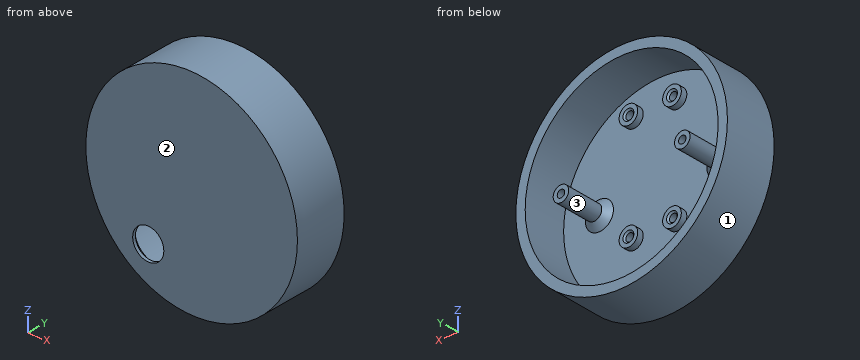
Autodesk Inventor part; units mm, degrees
ref_plane "YZ Plane" through (0, 0, 0) normal (1, 0, 0) x (0, 1, 0)
ref_plane "XZ Plane" through (0, 0, 0) normal (0, 1, 0) x (-1, 0, 0)
ref_plane "XY Plane" through (0, 0, 0) normal (0, 0, 1) x (1, 0, 0)
sketch "Sketch1" plane through (0, 0, 0) normal (0, 1, 0) x (-1, 0, 0)
  circle A0 centre (0, 0) radius 34
  dimension "d0" = 68
extrude "Extrusion1" add sketch "Sketch1" along normal blind 3
sketch "Sketch2" plane through (0, 3, 0) normal (0, 1, 0) x (1, 0, 0)
  circle A0 centre (0, 0) radius 34
  circle A1 centre (0, 0) radius 31
  dimension "d3" = 62
extrude "Extrusion2" add sketch "Sketch2" along normal blind 14
sketch "Sketch3" plane through (0, 3, 0) normal (0, 1, 0) x (1, 0, 0)
  circle A0 centre (0, 0) radius 31
  circle A1 centre (0, 0) radius 19.5
  line L0 (-19.5, 0) -> (19.5, 0)
  circle A2 centre (-19.5, 0) radius 1.2
  circle A3 centre (-19.5, 0) radius 2.5
  circle A4 centre (19.5, 0) radius 1.2
  circle A5 centre (19.5, 0) radius 2.5
  dimension "d6" = 39
  dimension "d7" = 2.4
  dimension "d8" = 5
  dimension "d9" = 2.4
  dimension "d10" = 5
extrude "Extrusion3" add sketch "Sketch3" along normal up to surface (14 mm away) contours A4 L0 A5 A1 | A1 A5 A4 | A1 A5 L0 A4 | A3 L0 A2 A1 | A1 A2 A3 | A1 A2 L0 A3
chamfer "Chamfer1" distance 2 angle 45 2 edges at (-22, 3, 0) (17, 3, 0)
sketch "Sketch4" plane through (0, 3, 0) normal (0, 1, 0) x (1, 0, 0)
  circle A0 centre (-13.9417, 19.5241) radius 5
  dimension "d16" = 10
extrude "Extrusion4" cut sketch "Sketch4" against normal blind 14
chamfer "Chamfer2" distance 2 angle 45 1 edges at (-18.9417, 3, -19.5241)
sketch "Sketch5" plane through (0, 3, 0) normal (0, 1, 0) x (1, 0, 0)
  line L0 (-8.5812, 13.9919) -> (11.4188, 13.9919)
  line L1 (11.4188, 13.9919) -> (11.4188, -26.0081)
  line L2 (11.4188, -26.0081) -> (-8.5812, -26.0081)
  line L3 (-8.5812, -26.0081) -> (-8.5812, 13.9919)
  circle A0 centre (-5.5812, 10.9919) radius 1.25
  circle A1 centre (-5.5812, 10.9919) radius 3
  circle A2 centre (8.4188, 10.9919) radius 1.25
  circle A3 centre (8.4188, 10.9919) radius 3
  circle A4 centre (8.4188, -23.0081) radius 1.25
  circle A5 centre (8.4188, -23.0081) radius 3
  circle A6 centre (-5.5812, -23.0081) radius 1.25
  circle A7 centre (-5.5812, -23.0081) radius 3
  dimension "d22" = 20
  dimension "d23" = 40
  dimension "d24" = 2.5
  dimension "d25" = 6
  dimension "d26" = 2.5
  dimension "d27" = 6
  dimension "d28" = 2.5
  dimension "d29" = 6
  dimension "d30" = 2.5
  dimension "d31" = 6
  dimension "d32" = 3
  dimension "d33" = 3
  dimension "d34" = 3
  dimension "d35" = 3
  dimension "d36" = 3
  dimension "d37" = 3
  dimension "d38" = 3
  dimension "d39" = 3
extrude "Extrusion5" add sketch "Sketch5" along normal blind 2 contours A1 | A3 | A7 | A5
sketch "Sketch6" plane through (-5.5812, 3, -10.9919) normal (0, 1, 0) x (1, 0, 0)
  circle A0 centre (0, 0) radius 1.25
  circle A1 centre (0, 0) radius 1.25
  circle A2 centre (14, 0) radius 1.25
  circle A3 centre (14, -34) radius 1.25
  circle A4 centre (0, -34) radius 1.25
  point P0 (5.5812, -10.9919)
extrude "Extrusion6" cut sketch "Sketch6" against normal blind 2
chamfer "Chamfer3" distance 0.5 angle 45 4 edges at (-6.8312, 5, -10.9919) (7.1688, 5, -10.9919) (-6.8312, 5, 23.0081) (7.1688, 5, 23.0081)
properties part number "obudowa - czujnik dymu"
The model under review builds one solid part; all positions refer to its coordinate system, in mm. Face numbers are marked on the shaded views. Round coordinates to 2 decimals unless told otherwise and drop trailing zeros. Loops run counter-clockwise (first coordinate to the right, second up) from the corner with the lowest first, then second, coordinate; pieces in that order, holes last. Notation, with made-up numbers: (-33.75, 37.25) -> (-16.75, 37.25) arc R10 ccw to (-16.75, 45.25) -> close; hole circle Ø10 at (-12, 89.5). An arc over 180 degrees is marked (long way). Answer as CSV lines item,"result".
1) To check wall thickness, follow line 1 along X through (y, z) = (7.5, 0); line 2 along X through (y, z) = (10, -2); line 3 along Z through (x, y) = (21.5, 16.25). State the ranges of each line that lie inside material, in increasing order. Write a range as from..to.
Geometry results:
line 1,"x = -34..-31, -22..-20.7, -18.3..-17, 17..18.3, 20.7..22, 31..34"
line 2,"x = -33.94..-30.94, -21..-18, 18..21, 30.94..33.94"
line 3,"z = -26.34..-22.33, -1.5..1.5, 22.33..26.34"
2) Add section B-B on z = -5.5. Write out the cut boundary in (x, y), plus the area to 3 significant figures.
Geometry results:
outline,"(-33.55, 0) -> (33.55, 0) -> (33.55, 17) -> (30.51, 17) -> (30.51, 3) -> (-30.51, 3) -> (-30.51, 17) -> (-33.55, 17) -> close"
area,"287 mm²"
3) Add section A-A on y = 6. Write out the cut boundary in (x, z).
Geometry results:
outline,"circle Ø68 at (0, 0); circle Ø5 at (-19.5, 0); circle Ø5 at (19.5, 0); hole circle Ø62 at (0, 0); hole circle Ø2.4 at (-19.5, 0); hole circle Ø2.4 at (19.5, 0)"
4) Add section C-C on y = 2. Write out the cut boundary in (x, z).
Geometry results:
outline,"circle Ø68 at (0, 0); hole circle Ø12 at (-13.94, -19.52); hole circle Ø2.5 at (-5.58, -10.99); hole circle Ø2.5 at (-5.58, 23.01); hole circle Ø2.5 at (8.42, -10.99); hole circle Ø2.5 at (8.42, 23.01)"
5) Draft analysis for pull direction X (two halves, no side actions). For the marked faces 1, 2 and 3, state which applies: pulls with the +X half, pulls with the -X half, needs draft (parallel to the pull), parting line crosses it, or undercut.
Geometry results:
face 1,"parting line crosses it"
face 2,"needs draft"
face 3,"undercut"
6) For P1, Ø0.7, axis at x = -19, z = 0, coming from the +Y side; P2, Ø8, axis at x = 4, y = 2, coming from the +Z side; P3, Ø5, axis at x = 7.5, z = -9.5, coming from the +Y side; P4, Ø8, axis at x = -13.94, z = -19.52, coming from the +Y side, all flat-tipped, find the tip position at first contact; note any pin that passes through.
Geometry results:
P1,"stops at y = 3"
P2,"stops at z = 34"
P3,"stops at y = 5"
P4,"passes through"
